```python
from build123d import *

# Parameters (mm, degrees)
BASE_EXTRUSION_DEPTH      = 7
BASE_EXTRUSION_DEPTH_BACK = 7
BOSS_EXTRU_4_DEPTH        = 19
BOSS_EXTRU_4_DEPTH_BACK   = 19
ESQUISSE8_R               = 5
BOSS_EXTRU_5_DEPTH        = 19
BOSS_EXTRU_5_DEPTH_BACK   = 19
ESQUISSE9_R               = 5
CHANFREIN2_SIZE           = 1


with BuildPart() as part:
    # Esquisse1 → Base-Extrusion (new, two sides: drawn at the far end of the back side and taken through both)
    with BuildSketch(Plane.XY.offset(-BASE_EXTRUSION_DEPTH_BACK)):
        with BuildLine():
            Line((-5.408326913, 9), (5.408326913, 9))
            ThreePointArc((5.408326913, 9), (7.424621202, 7.424621202), (9, 5.408326913))
            Line((9, 5.408326913), (9, -5.408326913))
            ThreePointArc((9, -5.408326913), (7.424621202, -7.424621202), (5.408326913, -9))
            Line((5.408326913, -9), (-5.408326913, -9))
            ThreePointArc((-5.408326913, -9), (-7.424621202, -7.424621202), (-9, -5.408326913))
            Line((-9, -5.408326913), (-9, 5.408326913))
            ThreePointArc((-9, 5.408326913), (-7.424621202, 7.424621202), (-5.408326913, 9))
        make_face()
    extrude(amount=BASE_EXTRUSION_DEPTH + BASE_EXTRUSION_DEPTH_BACK)

    # Esquisse8 → Boss.-Extru.4 (add, two sides: drawn at the far end of the back side and taken through both)
    with BuildSketch(Plane(origin=(0, 0, 0), x_dir=(1, 0, 0), z_dir=(0, 1, 0)).offset(-BOSS_EXTRU_4_DEPTH_BACK)):
        with Locations(Location((0, 0, 0), (0, 0, 90))):
            Circle(ESQUISSE8_R)
    extrude(amount=BOSS_EXTRU_4_DEPTH + BOSS_EXTRU_4_DEPTH_BACK)

    # Esquisse9 → Boss.-Extru.5 (add, two sides: drawn at the far end of the back side and taken through both)
    with BuildSketch(Plane(origin=(0, 0, 0), x_dir=(0, 0, -1), z_dir=(1, 0, 0)).offset(-BOSS_EXTRU_5_DEPTH_BACK)):
        with Locations(Location((0, 0, 0), (0, 0, 180))):
            Circle(ESQUISSE9_R)
    extrude(amount=BOSS_EXTRU_5_DEPTH + BOSS_EXTRU_5_DEPTH_BACK)

    # Chanfrein2
    chanfrein2_edges = [part.edges().sort_by_distance(p)[0] for p in [
        (0, 19, 5),
        (-19, 0, -5),
        (19, 0, -5),
        (0, -19, 5),
    ]]
    chamfer(chanfrein2_edges, length=CHANFREIN2_SIZE)


solid = part.part
```
CAD build for the part. Positions are in the model's coordinates, mm. A direction names the side the tool comes from. Coordinates: 2 decimals unless noted, no trailing zeros. Write each loop counter-clockwise with the first axis right and the second up, starting at its lowest first coordinate (ties: lowest second). Pieces come first, ordered by that corner, then holes.
(1) Flat gauge pins, fed straight in: pin 1 (4 mm diameter, centred on x = -13.5, z = 1, fed in from -Y); pin 2 (5 mm diameter, centred on x = -10, z = -1.5, fed in from +Y). Where does each tip first touch, or does it go through?
(2) Cut at D-D, the plane z = 5.5. List the corners of the cut face in (x, y).
(3) 3-axis set-ups, long thin cutter, end or side, ignore diameter. For faces 1 (the face through (5, -9, -2)), 2 (the face through (13, 0, -5)), 3 (the face through (-14, 0, -5)): which of +Z, -Z, +X, -X, +Y, -Y reach the whole face in a straight line?
(4) Cut at B-B, the plane x = 0. List the corners of the cut face in (y, z).
(5) Drill centre lines: probe 1 along X at (y, z) = (-5, -3.75); probe 2 along Y at (x, z) = (-6, 0.75); probe 3 along Y at (x, z) = (-9.5, 0.5). Where is each one in solid material? Low to high.
Geometry says:
1. pin 1: stops at y = -5
1. pin 2: stops at y = 7.35
2. outline: (-9, -5.41) arc R10.5 ccw to (-5.41, -9) - (5.41, -9) arc R10.5 ccw to (9, -5.41) - (9, 5.41) arc R10.5 ccw to (5.41, 9) - (-5.41, 9) arc R10.5 ccw to (-9, 5.41) - close
3. face 1: -Y
3. face 2: +X
3. face 3: -X
4. outline: (-19, -4) - (-18, -5) - (-9, -5) - (-9, -7) - (9, -7) - (9, -5) - (18, -5) - (19, -4) - (19, 4) - (18, 5) - (9, 5) - (9, 7) - (-9, 7) - (-9, 5) - (-18, 5) - (-19, 4) - close
5. probe 1: x = -9 to 9
5. probe 2: y = -8.62 to 8.62
5. probe 3: y = -4.97 to 4.97
